from build123d import *

# Parameters (mm, degrees)
SZKIC1_R                    = 5
DODANIE_WYCI_GNI_CIE1_DEPTH = 30
SZKIC1_3_R                  = 3
DODANIE_WYCI_GNI_CIE2_DEPTH = 20
ZAOKR_GLENIE1_R             = 5
DODANIE_WYCI_GNI_CIE3_DEPTH = 25


with BuildPart() as part:
    # Szkic1 → Dodanie-wyciągnięcie1 (new body)
    with BuildSketch(Plane.XY):
        Circle(SZKIC1_R)
    extrude(amount=DODANIE_WYCI_GNI_CIE1_DEPTH)

    # Szkic1<3> → Dodanie-wyciągnięcie2 (add)
    with BuildSketch(Plane.XY):
        Circle(SZKIC1_3_R)
    extrude(amount=-DODANIE_WYCI_GNI_CIE2_DEPTH)

    # Zaokrąglenie1
    zaokr_glenie1_edges = [part.edges().sort_by_distance(p)[0] for p in [
        (-5, 0, 30),
    ]]
    fillet(zaokr_glenie1_edges, radius=ZAOKR_GLENIE1_R)

    # Szkic3 → Dodanie-wyciągnięcie3 (add)
    with BuildSketch(Plane(origin=(0, 0, 0), x_dir=(-1, 0, 0), z_dir=(0, 0, -1))):
        with BuildLine():
            Line((2.5, -6.830127019), (2.5, -4.330127019))
            ThreePointArc((2.5, -4.330127019), (0, -5), (-2.5, -4.330127019))
            Line((-2.5, -4.330127019), (-2.5, -6.830127019))
            Line((-2.5, -6.830127019), (2.5, -6.830127019))
        make_face()
    extrude(amount=-DODANIE_WYCI_GNI_CIE3_DEPTH)


solid = part.part
The listing builds one solid part. Answer for the finished solid, in the listing's coordinates (mm). A direction names the side the tool comes from. Coordinates: 2 decimals unless noted, no trailing zeros. Write each loop counter-clockwise with the first axis right and the second up, starting at its lowest first coordinate (ties: lowest second). Pieces come first, ordered by that corner, then holes. Notation, with made-up numbers: (34, 34) - (53, 34) arc R5 cw to (53, 41) - close; hole circle Ø9 at (59.25, 89.25). An arc over 180 degrees is marked (long way). Return JSON: item names as keys, results as strings.
1. The part is cut by section A-A on y = 0. Determine the outline of the cut face in (x, z), then the cut area to 3 significant figures.
Final values:
{"outline": "(-5, 0) - (-3, 0) - (-3, -20) - (3, -20) - (3, 0) - (5, 0) - (5, 25) arc R5 ccw to (-5, 25) - close", "area": "409 mm^2"}
2. The part is cut by section C-C on z = -5.5. Determine the outline of the cut face in (x, y).
Final values:
{"outline": "circle Ø6 at (0, 0)"}
3. Each of these flat-tipped pins is pushed along its axis until it touches: pin 1 Ø1.3 at (x, y) = (-0.5, -6) entering from +Z; pin 2 Ø1.5 at (y, z) = (-2.5, 2) entering from +X; pin 3 Ø2 at (y, z) = (-5.5, 14.5) entering from +X. Where does it stop, or does it pass through?
Final values:
{"pin 1": "z = 25", "pin 2": "x = 4.68", "pin 3": "x = 2.5"}
4. Which of the six approach directions +Z, -Z, +X, -X, +Y, -Y give full straight-line access (tool end or side, diameter ignored) to faces 1 (the face through (-2.5, -6, 12)), 2 (the face through (0, 5, 12)), 3 (the face through (2.5, -6, 12)), 4 (the face through (-3, 0, -10))?
Final values:
{"face 1": "+Z, -Z, -X, -Y", "face 2": "+Z, -Z", "face 3": "+Z, -Z, +X, -Y", "face 4": "-Z"}
5. Consider line 1 along X through (y, z) = (-5, 19); line 2 along X through (y, z) = (4, 12.5); line 3 along Y through (x, z) = (-1.5, 3). Determine where each line is inside the solid, lowest interval first.
Final values:
{"line 1": "-2.5 to 2.5", "line 2": "-3 to 3", "line 3": "-6.83 to 4.77"}
6. The part is cut by section D-D on y = 2.25. Determine the outline of the cut face in (x, z), then the cut area to 3 significant figures.
Final values:
{"outline": "(-4.47, 0) - (-1.98, 0) - (-1.98, -20) - (1.98, -20) - (1.98, 0) - (4.47, 0) - (4.47, 25) arc R4.47 ccw to (-4.47, 25) - close", "area": "334 mm^2"}
7. The part is cut by section B-B on x = 0. Determine the outline of the cut face in (y, z), then the cut area to 3 significant figures.
Final values:
{"outline": "(-6.83, 0) - (-3, 0) - (-3, -20) - (3, -20) - (3, 0) - (5, 0) - (5, 25) arc R5 ccw to (-5, 25) - (-6.83, 25) - close", "area": "455 mm^2"}
